Print and shaded views of the part. All mm, measured from the part's lowest x, y and z. A direction names the side the tool comes from. Coordinates: 2 decimals unless noted, no trailing zeros. Order: outer loops, then holes, each group sorted by start corner. A loop starts at its lowest first (then second) coordinate and runs counter-clockwise, first axis right, second up. Notation, with made-up numbers: (-30.75, 14.25) -> (21.25, 14.25) arc R24 cw to (21.25, 40.25) -> close; hole circle Ø10 at (-12, 77.25). An arc over 180 degrees is marked (long way). Write item = value, one per line. Start each with the question number.
Q1. Flat gauge pins, fed straight in: pin 1 (2.5 mm diameter, centred on x = 12, y = 9, fed in from -Z); pin 2 (5 mm diameter, centred on x = 65, y = 4, fed in from -Z); pin 3 (8 mm diameter, centred on y = 20.5, z = 43.5, fed in from +X); pin 4 (4 mm diameter, centred on x = 12, y = 23, fed in from -Z). Where does each tip first touch, or does it go through?
Q2. Cut at B-B, the plane x = 100. List the corners of the cut face in (y, z), plus the area to 3 significant figures.
Q3. Wall check: line 1 (Y direction, x = 12, z = 1.05); line 2 (Y direction, x = 100, z = 50.05); line 3 (Z direction, x = 20, y = 22.5). Give the ranges that are in metal, low to high. Write a range as from..to.
Q4. 3-axis set-ups, long thin cutter, end or side, ignore diameter. For the marked faces 1, 2 and 3: which of +Z, -Z, +X, -X, +Y, -Y reach the whole face in a straight line?
Q5. Cut at D-D, the plane z = 18. List the corners of the cut face in (x, y).
Q6. Cut at A-A, the plane y = 16. List the corners of the cut face in (x, z), plus the area to 3 significant figures.
Q7. Cut at C-C, the plane y = 23. List the corners of the cut face in (x, z), plus the area to 3 significant figures.
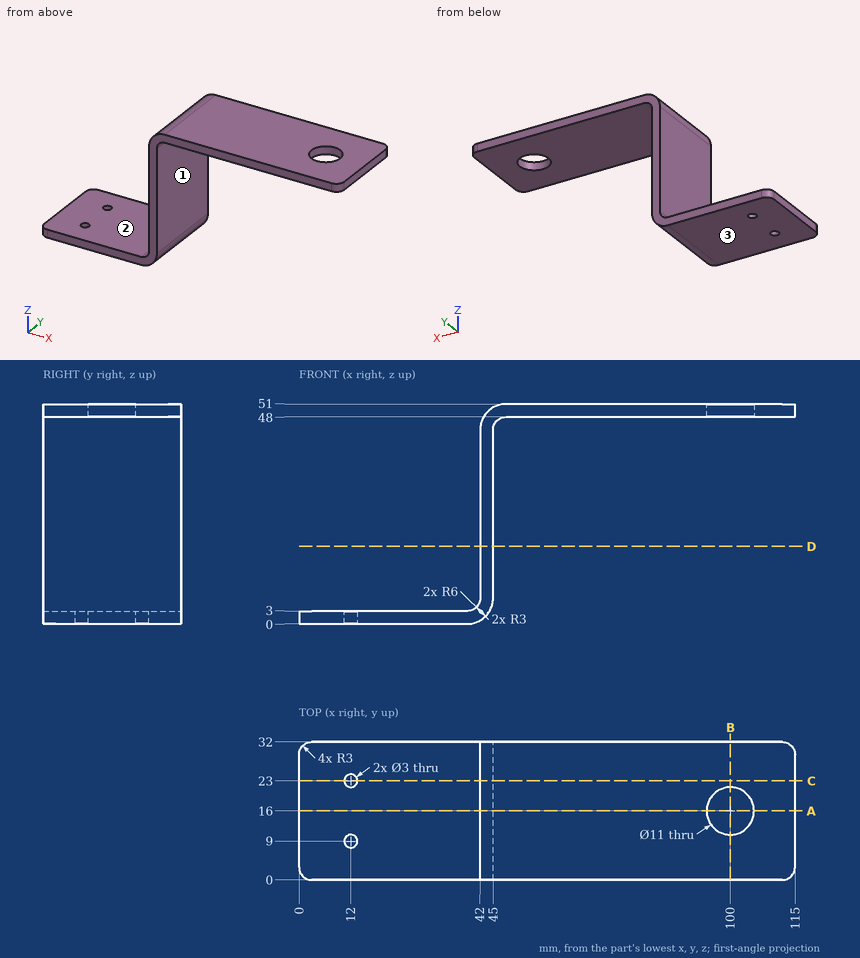
Here are the results:
q1.pin_1 = through
q1.pin_2 = 48
q1.pin_3 = 46.34
q1.pin_4 = 0
q2.outline = (0, 48) -> (10.5, 48) -> (10.5, 51) -> (0, 51) -> close; (21.5, 48) -> (32, 48) -> (32, 51) -> (21.5, 51) -> close
q2.area = 63.0 mm²
q3.line_1 = 0..7.5, 10.5..21.5, 24.5..32
q3.line_2 = 0..10.5, 21.5..32
q3.line_3 = 0..3
q4.face_1 = -Z, +X, +Y, -Y
q4.face_2 = +Z, -X, +Y, -Y
q4.face_3 = -Z, +X, -X, +Y, -Y
q5.outline = (42, 0) -> (45, 0) -> (45, 32) -> (42, 32) -> close
q6.outline = (0, 0) -> (39, 0) arc R6 ccw to (45, 6) -> (45, 45) arc R3 cw to (48, 48) -> (94.5, 48) -> (94.5, 51) -> (48, 51) arc R6 ccw to (42, 45) -> (42, 6) arc R3 cw to (39, 3) -> (0, 3) -> close; (105.5, 48) -> (115, 48) -> (115, 51) -> (105.5, 51) -> close
q6.area = 444 mm²
q7.outline = (0, 0) -> (10.5, 0) -> (10.5, 3) -> (0, 3) -> close; (13.5, 0) -> (39, 0) arc R6 ccw to (45, 6) -> (45, 45) arc R3 cw to (48, 48) -> (115, 48) -> (115, 51) -> (48, 51) arc R6 ccw to (42, 45) -> (42, 6) arc R3 cw to (39, 3) -> (13.5, 3) -> close
q7.area = 468 mm²
